Read the model definition and answer for the solid it produces. Units are mm, in the model's axes. A direction names the side the tool comes from. Coordinates: 2 decimals unless noted, no trailing zeros. Write each loop counter-clockwise with the first axis right and the second up, starting at its lowest first coordinate (ties: lowest second). Pieces come first, ordered by that corner, then holes. Notation, with made-up numbers: (-1, 73.25) - (43, 73.25) arc R27 cw to (43, 92.25) - close; hole circle Ø3 at (30, -21.75). An arc over 180 degrees is marked (long way). Use a Markdown table: item, result.
from build123d import *

# Parameters (mm, degrees)
SKETCH1_W                           = 20
SKETCH1_H                           = 19
BOSS_EXTRUDE1_DEPTH                 = 10
SKETCH2_R                           = 2.5
CUT_EXTRUDE1_DEPTH                  = 18.036725037
SKETCH3_R                           = 3.05
CUT_EXTRUDE2_DEPTH                  = 25.295061227
DI_METRO_DE_TALADRO_2_8_2_8_1_D     = 2.8
DI_METRO_DE_TALADRO_2_8_2_8_1_DEPTH = 14
DI_METRO_DE_TALADRO_2_8_2_8_1_TIP   = 0.841204867
TALADRO_ROSCADO_M31_REACH           = 22.387
TALADRO_ROSCADO_M31_BORE_R          = 1.25


with BuildPart() as part:
    # Sketch1 → Boss-Extrude1 (new body)
    with BuildSketch(Plane.XY):
        Rectangle(SKETCH1_W, SKETCH1_H)
    extrude(amount=BOSS_EXTRUDE1_DEPTH)

    # Sketch2 → Cut-Extrude1 (cut, through all)
    with BuildSketch(Plane(origin=(0, 0, 0), x_dir=(-1, 0, 0), z_dir=(0, 0, -1))):
        with Locations((0, -1.5)):
            Circle(SKETCH2_R)
    extrude(amount=-CUT_EXTRUDE1_DEPTH, mode=Mode.SUBTRACT)

    # Sketch3 → Cut-Extrude2 (cut, through all)
    with BuildSketch(Plane(origin=(10, 0, 0), x_dir=(0, 0, -1), z_dir=(1, 0, 0))):
        with Locations((-4.5, 5.25)):
            Circle(SKETCH3_R)
    extrude(amount=-CUT_EXTRUDE2_DEPTH, mode=Mode.SUBTRACT)

    # Diámetro de taladro Ø2.8 (2.8)1
    with Locations(Plane(origin=(10, 0, 0), x_dir=(0, 0, -1), z_dir=(1, 0, 0))):
        with Locations((-5, -6.5)):
            Hole(DI_METRO_DE_TALADRO_2_8_2_8_1_D / 2, depth=DI_METRO_DE_TALADRO_2_8_2_8_1_DEPTH)
            with Locations((0, 0, -(DI_METRO_DE_TALADRO_2_8_2_8_1_DEPTH + DI_METRO_DE_TALADRO_2_8_2_8_1_TIP / 2))):  # 118° drill point
                Cone(0, DI_METRO_DE_TALADRO_2_8_2_8_1_D / 2, DI_METRO_DE_TALADRO_2_8_2_8_1_TIP, mode=Mode.SUBTRACT)

    # Taladro roscado M31 bore → Taladro roscado M31 (cut, up to next)
    with BuildSketch(Plane(origin=(-2.648652683, -2.97524228, 10), x_dir=(1, 0, 0), z_dir=(0, 0, 1)), mode=Mode.PRIVATE) as taladro_roscado_m31_sk1:
        with Locations((9.648652683, 8.22524228)):
            Circle(TALADRO_ROSCADO_M31_BORE_R)
    taladro_roscado_m31_tool1 = extrude(taladro_roscado_m31_sk1.sketch, amount=-TALADRO_ROSCADO_M31_REACH, mode=Mode.PRIVATE) & part.part
    # Taladro roscado M31 bore → Taladro roscado M31 (cut, up to next)
    with BuildSketch(Plane(origin=(-2.648652683, -2.97524228, 10), x_dir=(1, 0, 0), z_dir=(0, 0, 1)), mode=Mode.PRIVATE) as taladro_roscado_m31_sk2:
        with Locations((9.648652683, -3.52475772)):
            Circle(TALADRO_ROSCADO_M31_BORE_R)
    taladro_roscado_m31_tool2 = extrude(taladro_roscado_m31_sk2.sketch, amount=-TALADRO_ROSCADO_M31_REACH, mode=Mode.PRIVATE) & part.part
    add(taladro_roscado_m31_tool1.solids().sort_by_distance((7, 5.25, 10))[0], mode=Mode.SUBTRACT)
    add(taladro_roscado_m31_tool2.solids().sort_by_distance((7, -6.5, 10))[0], mode=Mode.SUBTRACT)


solid = part.part
(1) The mould has two halves that part along Y. Classify faces 1 (the cylindrical face through (2.9, -6.44, 3.6)), 2 (the flat face through (0, 2, 0)), 3 (the flat face through (0, -9.5, 5)): pulls with the +Y half, pulls with the -Y half, needs draft (parallel to the pull), parting line crosses it, or undercut.
Report:
| item | result |
|---|---|
| face 1 | undercut |
| face 2 | needs draft |
| face 3 | pulls with the -Y half |
(2) Straight lines are drawn through the part: L1, parallel to Y at x = 6.75, z = 5; L2, parallel to Z at x = 5, y = -6.5; L3, parallel to Y at x = 7, z = 8.9. For each, find the intervals that lie inside material, in ascending order.
Report:
| item | result |
|---|---|
| L1 | y = -9.5 to -7.9, -5.1 to 2.24, 8.26 to 9.5 |
| L2 | z = 0 to 3.6, 6.4 to 10 |
| L3 | y = -9.5 to -7.75, -5.25 to 4, 6.5 to 9.5 |
(3) A cutting plane is placed at B-B, the plane y = 5.25. Write down the section's boundary in (x, z).
Report:
| item | result |
|---|---|
| outline | (-10, 0) - (10, 0) - (10, 1.45) - (-10, 1.45) - close; (-10, 7.55) - (5.75, 7.55) - (5.75, 10) - (-10, 10) - close; (8.25, 7.55) - (10, 7.55) - (10, 10) - (8.25, 10) - close |
(4) A cutting plane is placed at D-D, the plane y = 0.25. Write down the section's boundary in (x, z), and give its area (3 significant figures).
Report:
| item | result |
|---|---|
| outline | (-10, 0) - (-1.79, 0) - (-1.79, 10) - (-10, 10) - close; (1.79, 0) - (10, 0) - (10, 10) - (1.79, 10) - close |
| area | 164 mm² |
(5) A cutting plane is placed at A-A, the plane x = 0. Write down the section's boundary in (y, z), and give its area (3 significant figures).
Report:
| item | result |
|---|---|
| outline | (-9.5, 0) - (-4, 0) - (-4, 10) - (-9.5, 10) - close; (1, 0) - (9.5, 0) - (9.5, 10) - (1, 10) - close; hole circle Ø2.8 at (-6.5, 5); hole circle Ø6.1 at (5.25, 4.5) |
| area | 105 mm² |
(6) A cutting plane is placed at C-C, the plane z = 8. Write down the section's boundary in (x, y).
Report:
| item | result |
|---|---|
| outline | (-10, -9.5) - (10, -9.5) - (10, 9.5) - (-10, 9.5) - close; hole circle Ø5 at (0, -1.5); hole circle Ø2.5 at (7, -6.5); hole circle Ø2.5 at (7, 5.25) |
(7) For faces 4 (the flat face through (-10, 0, 5)), 5 (the cylindrical face through (6.84, 6.49, 8.66)), determine the directions among +Z, -Z, +X, -X, +Y, -Y from which every point of the face is accessible in a straight line to the end or side of a thin tool.
Report:
| item | result |
|---|---|
| face 4 | +Z, -Z, -X, +Y, -Y |
| face 5 | +Z |
